from build123d import *

# Parameters (mm, degrees)
CROQUIS1_W     = 500
CROQUIS1_H     = 500
EXTRUIR1_DEPTH = 500
CROQUIS2_R     = 115
EXTRUIR2_DEPTH = 40
REDONDEO1_R    = 20
VACIADO1_T     = -3
CROQUIS3_R     = 15
EXTRUIR3_DEPTH = 30


with BuildPart() as part:
    # Croquis1 → Extruir1 (new body)
    with BuildSketch(Plane(origin=(0, 0, 0), x_dir=(1, 0, 0), z_dir=(0, 1, 0))):
        Rectangle(CROQUIS1_W, CROQUIS1_H)
    extrude(amount=EXTRUIR1_DEPTH)

    # Croquis2 → Extruir2 (add)
    with BuildSketch(Plane(origin=(0, 500, 0), x_dir=(1, 0, 0), z_dir=(0, 1, 0))):
        with Locations(Location((0, 0, 0), (0, 0, 270))):
            Circle(CROQUIS2_R)
    extrude(amount=EXTRUIR2_DEPTH)

    # Redondeo1
    redondeo1_edges = [part.edges().sort_by_distance(p)[0] for p in [
        (250, 500, 0),
        (0, 500, -250),
        (0, 500, -115),
        (-250, 500, 0),
        (0, 0, -250),
        (250, 0, 0),
        (0, 0, 250),
        (-250, 0, 0),
        (0, 500, 250),
        (-250, 250, -250),
        (250, 250, -250),
        (250, 250, 250),
        (-250, 250, 250),
    ]]
    fillet(redondeo1_edges, radius=REDONDEO1_R)

    # Vaciado1
    vaciado1_openings = [part.faces().sort_by_distance(p)[0] for p in [
        (0, 540, 0),
    ]]
    offset(amount=VACIADO1_T, openings=vaciado1_openings, kind=Kind.INTERSECTION)

    # Croquis3 → Extruir3 (cut)
    with BuildSketch(Plane(origin=(0, 500, 0), x_dir=(1, 0, 0), z_dir=(0, 1, 0))):
        with Locations(Location((174.828263658, 188.220904974, 0), (0, 0, 270))):
            Circle(CROQUIS3_R)
    extrude(amount=-EXTRUIR3_DEPTH, mode=Mode.SUBTRACT)


solid = part.part
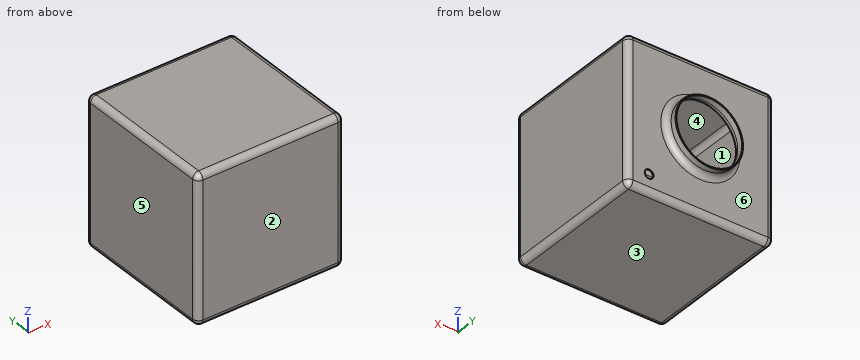
Verification items for the finished model (mm, model axes). Face numbers are marked on the shaded views. A direction names the side the tool comes from. Coordinates: 2 decimals unless noted, no trailing zeros. Order: outer loops, then holes, each group sorted by start corner. A loop starts at its lowest first (then second) coordinate and runs counter-clockwise, first axis right, second up. Notation, with made-up numbers: M 71.25,75.25 L 85.25,75.25 A16 cw 85.25,79.25 Z; hole C -36.5,76.25 d1. An arc over 180 degrees is marked long. One line per item, written item: value. Start each with the question number.
Item 1: Access from +Z, -Z, +X, -X, +Y, -Y to the whole of each face (thin tool, end or side, straight path). Record for the marked faces 5 and 6.
Item 2: Sectioned sample at C-C (z = 0). Enter the section's corners in (x, y), then the cut area to 3 significant figures.
Item 3: Sectioned sample at D-D (x = 0). Enter the section's corners in (y, z).
Item 4: Mould release check, pull along Y, two halves, no side actions. Record for the marked faces 1, 2, 3 and 4: released by +Y, released by -Y, zero draft, split by the parting line, or undercut.
Item 5: Scan lines: probe 1 along Z at (x, y) = (109.5, 246); probe 2 along Y at (x, z) = (-190.5, -171.5). Record each from-to range of solid material in increasing order.
Item 6: Sectioned sample at B-B (y = 317). Enter the section's corners in (x, z).
Item 7: Gauge pin test, flat ends, axial feed: pin 1 (8 mm diameter, centred on x = 26.5, z = 30.5, fed in from +Y); pin 2 (6 mm diameter, centred on x = -9.5, z = -140, fed in from +Y). Record the tip position at first contact, or that the pin passes through.
Item 8: Sectioned sample at A-A (x = -171). Enter the section's corners in (y, z), then the cut area to 3 significant figures.
Conclusion:
1. face 5: +Z, -Z, -X, +Y, -Y
1. face 6: +Y
2. outline: M -250,20 A20 ccw -230,0 L 230,0 A20 ccw 250,20 L 250,480 A20 ccw 230,500 L 135,500 A20 cw 115,520 L 115,540 L 112,540 L 112,520 A23 ccw 135,497 L 230,497 A17 cw 247,480 L 247,20 A17 cw 230,3 L -230,3 A17 cw -247,20 L -247,480 A17 cw -230,497 L -135,497 A23 ccw -112,520 L -112,540 L -115,540 L -115,520 A20 cw -135,500 L -230,500 A20 ccw -250,480 Z
2. area: 5,380 mm^2
3. outline: M 0,-230 A20 ccw 20,-250 L 480,-250 A20 ccw 500,-230 L 500,-135 A20 cw 520,-115 L 540,-115 L 540,-112 L 520,-112 A23 ccw 497,-135 L 497,-230 A17 cw 480,-247 L 20,-247 A17 cw 3,-230 L 3,230 A17 cw 20,247 L 480,247 A17 cw 497,230 L 497,135 A23 ccw 520,112 L 540,112 L 540,115 L 520,115 A20 cw 500,135 L 500,230 A20 ccw 480,250 L 20,250 A20 ccw 0,230 Z
4. face 1: undercut
4. face 2: released by -Y
4. face 3: zero draft
4. face 4: undercut
5. probe 1: z = -250 to -247, 247 to 250
5. probe 2: y = 0 to 3, 497 to 500
6. outline: M -250,-230 A20 ccw -230,-250 L 230,-250 A20 ccw 250,-230 L 250,230 A20 ccw 230,250 L -230,250 A20 ccw -250,230 Z; hole M -247,-230 A17 ccw -230,-247 L 230,-247 A17 ccw 247,-230 L 247,230 A17 ccw 230,247 L -230,247 A17 ccw -247,230 Z
7. pin 1: stops at y = 3
7. pin 2: stops at y = 500
8. outline: M 0,-230 A20 ccw 20,-250 L 480,-250 A20 ccw 500,-230 L 500,230 A20 ccw 480,250 L 20,250 A20 ccw 0,230 Z; hole M 3,-230 A17 ccw 20,-247 L 480,-247 A17 ccw 497,-230 L 497,230 A17 ccw 480,247 L 20,247 A17 ccw 3,230 Z
8. area: 5,870 mm^2
